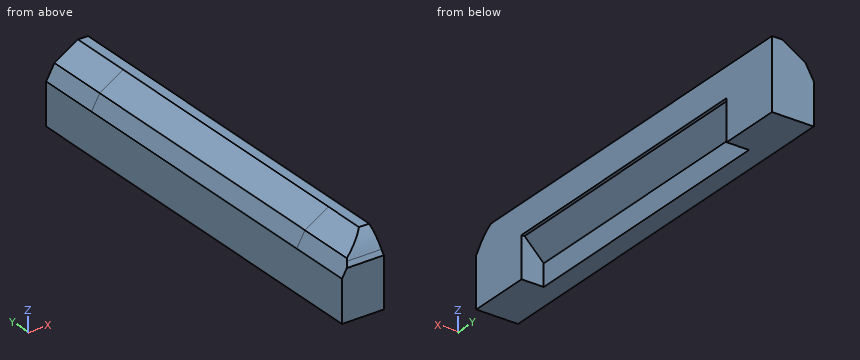
```python
from build123d import *

# Parameters (mm, degrees)
F1_DEPTH  = 7.45
F2_W      = 0.582146
F2_H      = 1.072485
F3_DEPTH  = 7.451
F4_SIZE   = 0.5
F5_SIZE   = 0.25
F7_DEPTH  = 1.643
F9_DEPTH  = 1.643
F11_W     = 10.736
F11_H     = 0.158
F12_DEPTH = 1.094878
F13_DEPTH = 1.094878


with BuildPart() as f1:
    # F0 (on Front) → F1 (new body)
    with BuildSketch(Plane.XZ):
        Polygon((0, 1.342732), (0, 0), (1.093878, 0), (1.093878, 1.085751), (1.093878, 2), align=None)
    extrude(amount=F1_DEPTH)

    # F2 (on face) → F3 (cut, through all)
    with BuildSketch(Plane.XZ.offset(7.45)):
        with Locations((0.802805, 0.536242)):
            Rectangle(F2_W, F2_H)
    extrude(amount=-F3_DEPTH, mode=Mode.SUBTRACT)

    # F4
    f4_edges = [f1.edges().sort_by_distance(p)[0] for p in [
        (0.511732, -3.725, 1.072485),
    ]]
    chamfer(f4_edges, length=F4_SIZE)

    # F5
    f5_edges = [f1.edges().sort_by_distance(p)[0] for p in [
        (0, -3.725, 1.342732),
    ]]
    chamfer(f5_edges, length=F5_SIZE)

    # F6 (on face) → F7 (join)
    with BuildSketch(Plane(origin=(0, 0, 0), x_dir=(-1, 0, 0), z_dir=(0, 1, 0))):
        Polygon((-0.214292, 1.471492), (-1.093878, 2), (-1.093878, 0), (0, 0), (0, 1.092732), align=None)
    extrude(amount=F7_DEPTH)

    # F8 (on face) → F9 (join)
    with BuildSketch(Plane.XZ.offset(7.45)):
        Polygon((1.093878, 0), (1.093878, 2), (0.214292, 1.471492), (0, 1.092732), (0, 0), align=None)
    extrude(amount=F9_DEPTH)

    # F11 (on face) → F12 (cut, through all)
    with BuildSketch(Plane.YZ.offset(1.093878)):
        with Locations((-3.725, 1.921)):
            Rectangle(F11_W, F11_H)
    extrude(amount=-F12_DEPTH, mode=Mode.SUBTRACT)

    # F10 (on face) → F13 (cut, through all)
    with BuildSketch(Plane.YZ.offset(1.093878)):
        with BuildLine():
            Line((-9.093, 2), (-9.093, 1.31302))
            Line((-9.093, 1.31302), (-9.009582, 1.421623))
            ThreePointArc((-9.009582, 1.421623), (-8.629245, 1.79858), (-8.133078, 2))
            Line((-8.133078, 2), (-9.093, 2))
        make_face()
        with BuildLine():
            ThreePointArc((-7.6235, 2), (-7.878289, 2.024017), (-8.133078, 2))
            Line((-8.133078, 2), (-7.6235, 2))
        make_face()
    extrude(amount=-F13_DEPTH, mode=Mode.SUBTRACT)


solid = f1.part
```
Can you work these out from the model? Positions are in its coordinate system, mm. Give positions to 0.01 mm unless a question says otherwise; leave off trailing zeros. Write each loop counter-clockwise with the first axis right and the second up, starting at its lowest first coordinate (ties: lowest second). Pieces come first, ordered by that corner, then holes. Notation, with made-up numbers: (-17.75, 36.5) -> (26.25, 36.5) arc R34 cw to (26.25, 67.5) -> close; hole circle Ø4 at (72.5, 47). An arc over 180 degrees is marked (long way). One line per item, written item: value.
Q1. Please list where these lines run through material, in increasing order: line 1 (Y direction, x = 0.95, z = 0.75); line 2 (X direction, y = -4.5, z = 0.45); line 3 (X direction, y = -5.25, z = 0.9). Write a range as [from, to].
Results found:
line 1: y = [-9.09, -7.45], [0, 1.64]
line 2: x = [0, 0.51]
line 3: x = [0, 0.84]
Q2. Imagine slicing it at A-A on y = 1.25. Please give me the cut outline in (x, z), and give its area (3 significant figures).
Results found:
outline: (0, 0) -> (1.09, 0) -> (1.09, 1.84) -> (0.83, 1.84) -> (0.21, 1.47) -> (0, 1.09) -> close
area: 1.78 mm^2
Q3. Imagine slicing it at D-D on y = -1.5. Please give me the cut outline in (x, z).
Results found:
outline: (0, 0) -> (0.51, 0) -> (0.51, 0.57) -> (1.01, 1.07) -> (1.09, 1.07) -> (1.09, 1.84) -> (0.83, 1.84) -> (0.21, 1.47) -> (0, 1.09) -> close
Q4. For P1, Ø0.6, axis at y = -3, z = 0, coming from the +X side, with a flat end and sliding along its axis, tell me the tip position at first contact or that it passes through.
Results found:
P1: stops at x = 0.51
Q5. Imagine slicing it at C-C on z = 0.8. Please give me the cut outline in (x, y).
Results found:
outline: (0, -9.09) -> (1.09, -9.09) -> (1.09, -7.45) -> (0.74, -7.45) -> (0.74, 0) -> (1.09, 0) -> (1.09, 1.64) -> (0, 1.64) -> close
Q6. Imagine slicing it at B-B on x = 0.6. Please give me the cut outline in (y, z).
Results found:
outline: (-9.09, 0) -> (-7.45, 0) -> (-7.45, 0.66) -> (0, 0.66) -> (0, 0) -> (1.64, 0) -> (1.64, 1.7) -> (-8.76, 1.7) arc R1.36 ccw to (-9.01, 1.42) -> (-9.09, 1.31) -> close
